Input: part model. Units: mm. Frame: model coordinates. Face numbers are marked on the shaded views. A direction names the side the tool comes from. Round coordinates to 2 decimals unless told otherwise and drop trailing zeros. Loops run counter-clockwise (first coordinate to the right, second up) from the corner with the lowest first, then second, coordinate; pieces in that order, holes last. Notation, with made-up numbers: (76.5, 44) -> (115.5, 44) arc R19 cw to (115.5, 70) -> close; hole circle Ø4 at (1.5, 49). An arc over 180 degrees is marked (long way). Answer as a JSON object with one key per item and string values. Group by question number.
Item 1: Section query B-B on x = -12.6. Return loops of the section in (y, z), and give its area (3 significant figures).
Item 2: Section query C-C on z = 10.25. Return loops of the section in (x, y), and give its area (3 significant figures).
Item 3: Section query D-D on x = -3. Return loops of the section in (y, z).
Item 4: Material intervals for line 1 (X direction, y = -0.75, z = 14.5); line 2 (Z direction, x = 4, y = 3.75); line 3 (Z direction, x = -17.5, y = -1), sorted ascending. Write a range as [from, to].
Item 5: Set-up query: the marked faces 1 and 2. Return all of +Z, -Z, +X, -X, +Y, -Y with unobstructed straight access to the full face (end or side cutting, diameter ignored); none if empty.
Item 6: Section query A-A on y = -0.35. Return loops of the section in (x, z), and give its area (3 significant figures).
Item 7: Pin query (flat end, axial travel): pin 1 (6 mm diameter, centred on x = -11, y = -5, fed in from -Z); pin 2 (6 mm diameter, centred on x = -5.5, y = -7.5, fed in from +Z); pin 3 (1.6 mm diameter, centred on y = -9, z = -1, fed in from -X); pin 4 (4 mm diameter, centred on x = 4, z = 12, fed in from +Y). Return the tip coordinate at first contact, or that it passes through.
from build123d import *

# Parameters (mm, degrees)
SKETCH1_W           = 46
SKETCH1_H           = 20.5
BOSS_EXTRUDE1_DEPTH = 3.3
SKETCH2_R           = 8.4
BOSS_EXTRUDE2_DEPTH = 12
SKETCH3_W           = 10.3
SKETCH3_H           = 2.54
BOSS_EXTRUDE3_DEPTH = 2


with BuildPart() as part:
    # Sketch1 → Boss-Extrude1 (new body)
    with BuildSketch(Plane.XY):
        Rectangle(SKETCH1_W, SKETCH1_H)
    extrude(amount=BOSS_EXTRUDE1_DEPTH)

    # Sketch2 → Boss-Extrude2 (add)
    with BuildSketch(Plane.XY.offset(3.3)):
        with Locations(Location((-12.6, -0.35, 0), (0, 0, 180))):
            Circle(SKETCH2_R)
        with Locations(Location((12.6, -0.35, 0), (0, 0, 180))):
            Circle(SKETCH2_R)
    extrude(amount=BOSS_EXTRUDE2_DEPTH)

    # Sketch3 → Boss-Extrude3 (add)
    with BuildSketch(Plane(origin=(0, 0, 0), x_dir=(-1, 0, 0), z_dir=(0, 0, -1))):
        with Locations((0, -8.98)):
            Rectangle(SKETCH3_W, SKETCH3_H)
    extrude(amount=BOSS_EXTRUDE3_DEPTH)


solid = part.part
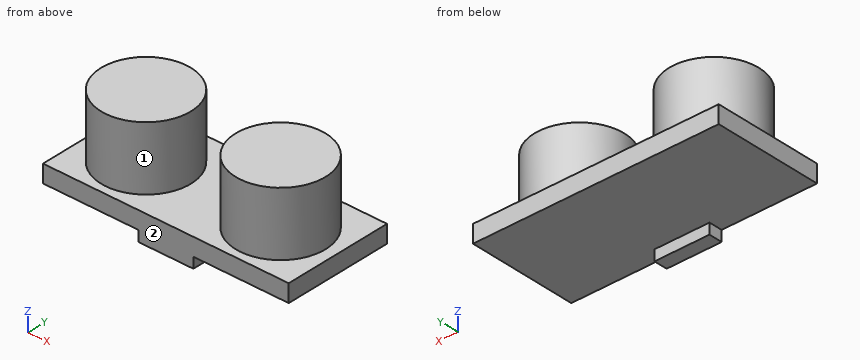
Solved:
{
 "1": {"outline": "(-10.25, 0) -> (10.25, 0) -> (10.25, 3.3) -> (8.05, 3.3) -> (8.05, 15.3) -> (-8.75, 15.3) -> (-8.75, 3.3) -> (-10.25, 3.3) -> close", "area": "269 mm²"},
 "2": {"outline": "circle Ø16.8 at (-12.6, -0.35); circle Ø16.8 at (12.6, -0.35)", "area": "443 mm²"},
 "3": {"outline": "(-10.25, -2) -> (-7.71, -2) -> (-7.71, 0) -> (10.25, 0) -> (10.25, 3.3) -> (-10.25, 3.3) -> close"},
 "4": {"line 1": "[-20.99, -4.21], [4.21, 20.99]", "line 2": "[0, 3.3]", "line 3": "[0, 15.3]"},
 "5": {"face 1": "+Z", "face 2": "+Z, -Z, +X, -X, -Y"},
 "6": {"outline": "(-23, 0) -> (23, 0) -> (23, 3.3) -> (21, 3.3) -> (21, 15.3) -> (4.2, 15.3) -> (4.2, 3.3) -> (-4.2, 3.3) -> (-4.2, 15.3) -> (-21, 15.3) -> (-21, 3.3) -> (-23, 3.3) -> close", "area": "555 mm²"},
 "7": {"pin 1": "z = 0", "pin 2": "z = 15.3", "pin 3": "x = -5.15", "pin 4": "y = 4.85"}
}
